The listing builds one solid part. Answer for the finished solid, in the listing's coordinates (mm). A direction names the side the tool comes from. Give positions to 0.01 mm unless a question says otherwise; leave off trailing zeros. Write each loop counter-clockwise with the first axis right and the second up, starting at its lowest first coordinate (ties: lowest second). Pieces come first, ordered by that corner, then holes. Notation, with made-up numbers: (70.25, 31.5) - (74.25, 31.5) arc R7 cw to (74.25, 37.5) - close; hole circle Ø6 at (27, -36.75). An arc over 180 degrees is marked (long way). Answer in a Markdown table with one row per item. Add a question column.
from build123d import *

# Parameters (mm, degrees)
BOSS_EXTRUDE1_DEPTH = 240
SKETCH2_W           = 70
SKETCH2_H           = 25
SKETCH2_W_2         = 29.546106777
SKETCH2_H_2         = 35
SKETCH2_R           = 12.5
BOSS_EXTRUDE2_DEPTH = 3
SKETCH3_R           = 9
BOSS_EXTRUDE3_DEPTH = 20
CHAMFER1_SIZE2      = 4.171137574
CHAMFER1_SIZE       = 3.5
SKETCH4_W           = 23.546106777
SKETCH4_H           = 29
BOSS_EXTRUDE4_DEPTH = 4
CUT_EXTRUDE1_DEPTH  = 27
SKETCH6_W           = 12
SKETCH6_H           = 19
BOSS_EXTRUDE5_DEPTH = 1


with BuildPart() as part:
    # Sketch1 → Boss-Extrude1 (new body)
    with BuildSketch(Plane(origin=(0, 0, 0), x_dir=(0, 0, -1), z_dir=(1, 0, 0))):
        Polygon((0, 0), (-66.758331831, 0), (-66.758331831, 10), (-32.219272119, 44.539059712), (93.241668169, 44.539059712), (93.241668169, 0), align=None)
    extrude(amount=BOSS_EXTRUDE1_DEPTH)

    # Sketch2 → Boss-Extrude2 (add)
    with BuildSketch(Plane(origin=(0, 38.379165915, 38.379165915), x_dir=(1, 0, 0), z_dir=(0, 0.7071067811865298, 0.7071067811865652))):
        with Locations((160.181803508, -15.788594651)):
            Rectangle(SKETCH2_W, SKETCH2_H)
        with Locations((27.103479103, -16.134201326)):
            Rectangle(SKETCH2_W_2, SKETCH2_H_2)
        with Locations(Location((77.833586966, -15.734201326, 0), (0, 0, 90))):
            Circle(SKETCH2_R)
    extrude(amount=BOSS_EXTRUDE2_DEPTH)

    # Sketch3 → Boss-Extrude3 (add)
    with BuildSketch(Plane(origin=(0, 40.500486259, 40.500486259), x_dir=(1, 0, 0), z_dir=(0, 0.7071067811865298, 0.7071067811865652))):
        with Locations(Location((77.833586966, -15.734201326, 0), (0, 0, 90))):
            Circle(SKETCH3_R)
    extrude(amount=BOSS_EXTRUDE3_DEPTH)

    # Chamfer1
    chamfer1_edges = [part.edges().sort_by_distance(p)[0] for p in [
        (77.833586966, 23.010764774, 57.990207744),
    ]]
    chamfer1_side = [part.faces().sort_by_distance(p)[0] for p in [
        (77.833586966, 22.961267299, 58.039705219),
    ]]
    chamfer(chamfer1_edges, length=CHAMFER1_SIZE - 0.0001, length2=CHAMFER1_SIZE2 - 0.0001, reference=chamfer1_side[0])  # a hair under: the kernel refuses the full size

    # Sketch4 → Boss-Extrude4 (add)
    with BuildSketch(Plane(origin=(0, 40.500486259, 40.500486259), x_dir=(1, 0, 0), z_dir=(0, 0.7071067811865298, 0.7071067811865652))):
        with Locations((27.103479102, -16.134201326)):
            Rectangle(SKETCH4_W, SKETCH4_H)
    extrude(amount=BOSS_EXTRUDE4_DEPTH)

    # Sketch5 → Cut-Extrude1 (cut)
    with BuildSketch(Plane.ZY.offset(-15.330425714)):
        with BuildLine():
            Line((44.484468223, 42.173358544), (48.455235169, 36.745535854))
            ThreePointArc((48.455235169, 36.745535854), (53.310708919, 31.055931968), (58.960608868, 26.154315063))
            Line((58.960608868, 26.154315063), (64.990564878, 21.66726189))
            Line((64.990564878, 21.66726189), (44.484468223, 42.173358544))
        make_face()
    extrude(amount=-CUT_EXTRUDE1_DEPTH, mode=Mode.SUBTRACT)

    # Sketch6 → Boss-Extrude5 (add)
    with BuildSketch(Plane(origin=(0, 40.500486259, 40.500486259), x_dir=(1, 0, 0), z_dir=(0, 0.7071067811865298, 0.7071067811865652))):
        with Locations((134.181803508, -15.788594651)):
            Rectangle(SKETCH6_W, SKETCH6_H)
        with Locations((149.181803508, -15.788594651)):
            Rectangle(SKETCH6_W, SKETCH6_H)
        with Locations((164.181803508, -15.788594651)):
            Rectangle(SKETCH6_W, SKETCH6_H)
    extrude(amount=BOSS_EXTRUDE5_DEPTH)


solid = part.part
1. The mould has two halves that part along Z. Classify faces 6 (the face through (118, 44.539, -30)), 7 (the face through (86.785, 30.775, 55.838)), 8 (the face through (26.94, 39.5, 46.44)): +Z half, -Z half, draft (parallel to the pull), parting line (faces both ways), or undercut.
2. Section A-A (x = 166) is taken. Give the vertices of the cut face in (y, z), and give its area (3 significant figures).
3. Section D-D (x = 26.5) is taken. Give the vertices of the cut face in (y, z), and give its area (3 significant figures).
4. Straight lines are drawn through the part: L1, parallel to Z at x = 28, y = 41; L2, parallel to Y at x = 204, z = 38.5; L3, parallel to Y at x = 40, z = -1. For each, find the intervals that lie inside material, in ascending order. Write a range as [from, to].
5. Given pin 1 Ø4 at (y, z) = (27.5, 54) entering from +X; pin 2 Ø5 at (x, y) = (104.5, 41) entering from +Z; pin 3 Ø8 at (y, z) = (33, 54) entering from -X, each flat-ended and moving along its own axis, determine where each tip first touches the part or whether it passes through.
6. Section C-C (z = 18) is taken. Give the vertices of the cut face in (x, y).
7. A tool of negligible diameter and unlimited length cuts with its end or side. For faces 1 (the face through (118, 23, -93.242)), 2 (the face through (170.182, 30, 52)), 3 (the face through (15.33, 30, 53)), 4 (the face through (240, 23, -14)), 5 (the face through (140.182, 30, 52)), from which of +Z, -Z, +X, -X, +Y, -Y can it reach the whole face along a straight path? Write none if from no direction.
8. Section B-B (y = 7.5) is taken. Give the vertices of the cut face in (x, z), and give its area (3 significant figures).
Geometry check:
| question | item | result |
|---|---|---|
| 1 | face 6 | draft |
| 1 | face 7 | undercut |
| 1 | face 8 | +Z half |
| 2 | outline | (0, -93.24) - (44.54, -93.24) - (44.54, 32.22) - (36.05, 40.7) - (38.18, 42.83) - (36.05, 44.95) - (36.76, 45.65) - (23.33, 59.09) - (22.62, 58.38) - (20.5, 60.5) - (18.38, 58.38) - (10, 66.76) - (0, 66.76) - close |
| 2 | area | 6,620 mm² |
| 3 | outline | (0, -93.24) - (44.54, -93.24) - (44.54, 32.22) - (39.34, 37.41) - (41.47, 39.53) - (39.34, 41.66) - (42.17, 44.48) - (36.75, 48.46) arc R50 cw to (26.15, 58.96) - (21.67, 64.99) - (18.84, 62.16) - (16.72, 64.28) - (14.6, 62.16) - (10, 66.76) - (0, 66.76) - close |
| 3 | area | 6,720 mm² |
| 4 | L1 | [-93.24, 35.76], [39.07, 40], [43.31, 45.34] |
| 4 | L2 | [0, 38.26] |
| 4 | L3 | [0, 44.54] |
| 5 | pin 1 | x = 195.18 |
| 5 | pin 2 | z = 38.26 |
| 5 | pin 3 | x = 15.33 |
| 6 | outline | (0, 0) - (240, 0) - (240, 44.54) - (0, 44.54) - close |
| 7 | face 1 | -Z, +X, -X, +Y, -Y |
| 7 | face 2 | +Z, +X, +Y |
| 7 | face 3 | +Z, -X, +Y |
| 7 | face 4 | +Z, -Z, +X, +Y, -Y |
| 7 | face 5 | +Z, +Y |
| 8 | outline | (0, -93.24) - (240, -93.24) - (240, 66.76) - (0, 66.76) - close |
| 8 | area | 38,400 mm² |
